Autodesk Inventor part; units mm, degrees
ref_plane "YZ Plane" through (0, 0, 0) normal (1, 0, 0) x (0, 1, 0)
ref_plane "XZ Plane" through (0, 0, 0) normal (0, 1, 0) x (-1, 0, 0)
ref_plane "XY Plane" through (0, 0, 0) normal (0, 0, 1) x (1, 0, 0)
sketch "Sketch1" plane through (0, 0, 0) normal (0, 1, 0) x (-1, 0, 0)
  line L0 (0.32, -0.32) -> (-0.32, -0.32)
  line L1 (-0.32, -0.32) -> (-0.32, 0.32)
  line L2 (-0.32, 0.32) -> (0.32, 0.32)
  line L3 (0.32, 0.32) -> (0.32, -0.32)
  line L4 (0.32, -0.32) -> (-0.32, 0.32) construction
  line L5 (-0.32, -0.32) -> (0.32, 0.32) construction
  point P0 (0, 0)
  dimension "d0" = 0.64
  dimension "d1" = 0.64
extrude "Extrusion1" add sketch "Sketch1" along normal blind 14.0176
chamfer "Chamfer1" distance 0.155 angle 45 8 edges at (0.32, 14.0176, 0) (0, 14.0176, -0.32) (0, 14.0176, 0.32) (-0.32, 14.0176, 0) (0.32, 0, 0) (0, 0, -0.32) (0, 0, 0.32) (-0.32, 0, 0)
sketch "Sketch2" plane through (-0.32, 0.155, 0.32) normal (0, 0, 1) x (1, 0, 0)
  line L0 (-0.9237, 9.6188) -> (1.8536, 9.6188)
  point P0 (0.32, -0.155)
  dimension "d7" = 9.7738
bend part "Bend Part1" radius 1 angle 90 line through (-1.2437, 9.7738, 0.32) along (1, 0, 0) centre toward (0, 0, 1) moving side (0, 1, 0) both sides no
properties part number "PinRight2" material "Gold"
Geometry: final body of the model. Coordinates: model frame, mm. Coordinates: 2 decimals unless noted, no trailing zeros. Write each loop counter-clockwise with the first axis right and the second up, starting at its lowest first coordinate (ties: lowest second). Pieces come first, ordered by that corner, then holes. Notation, with made-up numbers: M 30,20 L 60,20 A27 ccw 60,45 Z; hole C 30,19.5 d3. An arc over 180 degrees is marked long. Use CSV: the item, a comma, the result in double quotes. Start each with the question number.
1. Ray query, probe 1 along Y at (x, z) = (0.2, 1.25); probe 2 along Z at (x, y) = (-0.15, 5.75); probe 3 along Y at (x, z) = (0.05, 0.2) (3 decimals). Return the intervals inside material, ascending.
2. Cut plane A-A on x = 0.05. Return the cut outline in (y, z) (3 decimals).
3. Cut plane B-B on z = 3.7. Return the cut outline in (x, y).
4. Cut plane C-C on y = 6.75. Return the cut outline in (x, z), plus the area to 3 significant figures.
Entries:
1,probe 1,"10.77 to 11.41"
1,probe 2,"-0.32 to 0.32"
1,probe 3,"0.035 to 10.972"
2,outline,"M 0,-0.165 L 0.155,-0.32 L 9.774,-0.32 A1.64 ccw 11.414,1.32 L 11.414,3.838 L 11.259,3.993 L 10.929,3.993 L 10.774,3.838 L 10.774,1.32 A1 cw 9.774,0.32 L 0.155,0.32 L 0,0.165 Z"
3,outline,"M -0.32,10.77 L 0.32,10.77 L 0.32,11.41 L -0.32,11.41 Z"
4,outline,"M -0.32,-0.32 L 0.32,-0.32 L 0.32,0.32 L -0.32,0.32 Z"
4,area,"0.410 mm²"
